from build123d import *

# Parameters (mm, degrees)
SKETCH_1_W          = 6
SKETCH_1_H          = 6
EXTRUDE_1_DEPTH     = 21
SKETCH_2_R          = 1.5
CUT_EXTRUDE_1_DEPTH = 21
SKETCH_3_R          = 1.5
CUT_EXTRUDE_2_DEPTH = 21


with BuildPart() as part:
    # 草图1 → 凸台-拉伸1 (new body)
    with BuildSketch(Plane.XY):
        Rectangle(SKETCH_1_W, SKETCH_1_H)
    extrude(amount=EXTRUDE_1_DEPTH)

    # 草图2 → 切除-拉伸1 (cut)
    with BuildSketch(Plane.ZY.offset(3)):
        with Locations((3, 0)):
            Circle(SKETCH_2_R)
        with Locations((13, 0)):
            Circle(SKETCH_2_R)
    extrude(amount=-CUT_EXTRUDE_1_DEPTH, mode=Mode.SUBTRACT)

    # 草图3 → 切除-拉伸2 (cut)
    with BuildSketch(Plane(origin=(0, 3, 0), x_dir=(1, 0, 0), z_dir=(0, 1, 0))):
        with Locations((0.02150406, -18)):
            Circle(SKETCH_3_R)
        with Locations((0, -8)):
            Circle(SKETCH_3_R)
    extrude(amount=-CUT_EXTRUDE_2_DEPTH, mode=Mode.SUBTRACT)


solid = part.part
Work out the finished part from the listing and answer in its coordinate system (mm). Give positions to 0.01 mm unless a question says otherwise; leave off trailing zeros. Loops run counter-clockwise (first coordinate to the right, second up) from the corner with the lowest first, then second, coordinate; pieces in that order, holes last. Notation, with made-up numbers: (0, 63.5) -> (32, 63.5) arc R5 ccw to (32, 71.5) -> close; hole circle Ø4 at (-36, 49). An arc over 180 degrees is marked (long way). Use a Markdown table: item, result. Add a question column.
1) Consider line 1 along Y through (x, z) = (1.25, 3); line 2 along Z through (x, y) = (-0.8, 1.35); line 3 along Z through (x, y) = (0, 1.8). Determine where each line is inside the solid, lowest interval first.
2) The part is cut by section B-B, the plane z = 13. Determine the outline of the cut face in (x, y).
3) The part is cut by section A-A, the plane y = -1.2. Determine the outline of the cut face in (x, z), plus the area to 3 significant figures.
4) The part is cut by section D-D, the plane y = 2.3. Determine the outline of the cut face in (x, z).
5) The part is cut by section C-C, the plane x = 1.05. Determine the outline of the cut face in (y, z).
6) For a pull along Z with two mould halves and no side action, classify faces 1 (the flat face through (0, 0, 21)), 2 (the flat face through (0, 0, 0)), 3 (the cylindrical face through (-0.325, 0.042, 9.464)) as +Z half, -Z half, draft (parallel to the pull), parting line (faces both ways), or undercut.
Reported:
| question | item | result |
|---|---|---|
| 1 | line 1 | y = -3 to -1.5, 1.5 to 3 |
| 1 | line 2 | z = 0 to 2.35, 3.65 to 6.73, 9.27 to 12.35, 13.65 to 16.74, 19.26 to 21 |
| 1 | line 3 | z = 0 to 6.5, 9.5 to 16.5, 19.5 to 21 |
| 2 | outline | (-3, -3) -> (3, -3) -> (3, -1.5) -> (-3, -1.5) -> close; (-3, 1.5) -> (3, 1.5) -> (3, 3) -> (-3, 3) -> close |
| 3 | outline | (-3, 0) -> (3, 0) -> (3, 2.1) -> (-3, 2.1) -> close; (-3, 3.9) -> (3, 3.9) -> (3, 12.1) -> (-3, 12.1) -> close; (-3, 13.9) -> (3, 13.9) -> (3, 21) -> (-3, 21) -> close; hole circle Ø3 at (0, 8); hole circle Ø3 at (0.02, 18) |
| 3 | area | 90.3 mm^2 |
| 4 | outline | (-3, 0) -> (3, 0) -> (3, 21) -> (-3, 21) -> close; hole circle Ø3 at (0, 8); hole circle Ø3 at (0.02, 18) |
| 5 | outline | (-3, 0) -> (3, 0) -> (3, 6.93) -> (-3, 6.93) -> close; (-3, 9.07) -> (3, 9.07) -> (3, 16.91) -> (-3, 16.91) -> close; (-3, 19.09) -> (3, 19.09) -> (3, 21) -> (-3, 21) -> close; hole circle Ø3 at (0, 3); hole circle Ø3 at (0, 13) |
| 6 | face 1 | +Z half |
| 6 | face 2 | -Z half |
| 6 | face 3 | undercut |
